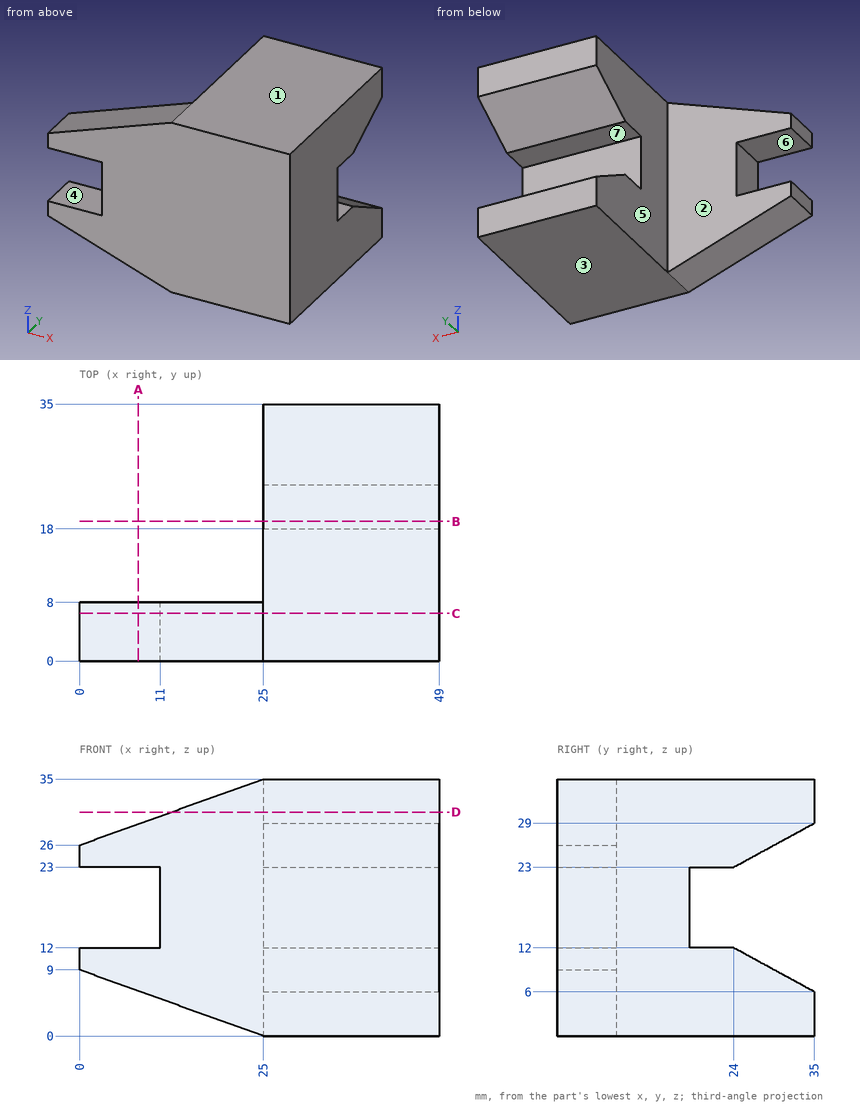
The drawing under review shows one solid part. Ordinate dimensions are in mm from its lowest x, y, z. A direction names the side the tool comes from. Coordinates: 2 decimals unless noted, no trailing zeros. Loops run counter-clockwise (first coordinate to the right, second up) from the corner with the lowest first, then second, coordinate; pieces in that order, holes last.
Item 1: Wall thickness on L1, parallel to Z at x = 30, y = 19; L2, parallel to Y at x = 9, z = 23.5; L3, parallel to X at y = 11.5, z = 2: over which ranges is each line inside the solid? List them lowest first.
Completed:
L1: z = 0 to 12, 23 to 35
L2: y = 0 to 8
L3: x = 25 to 49
Item 2: Add section C-C (y = 6.5). Write out the cut boundary in (x, z), and give its area (3 significant figures).
Completed:
outline: (0, 9) - (25, 0) - (49, 0) - (49, 35) - (25, 35) - (0, 26) - (0, 23) - (11, 23) - (11, 12) - (0, 12) - close
area: 1,370 mm2
Item 3: For the marked faces 5, 6 and 7, list the 3-axis set-ups (+Z, -Z, +X, -X, +Y, -Y) from which the entire face can be reached by the end or side of a thin tool; tool diameter is ignored.
Completed:
face 5: +Z, -Z, -X, +Y
face 6: -X, +Y, -Y
face 7: +X, -X, +Y
Item 4: Add section D-D (z = 30.5). Write out the cut boundary in (x, y).
Completed:
outline: (12.5, 0) - (49, 0) - (49, 35) - (25, 35) - (25, 8) - (12.5, 8) - close
Item 5: Clearance check with flat-ended pins moving along their axes: pin 1 (12 mm diameter, centred on y = 27.5, z = 20.5, fed in from -X); pin 2 (2 mm diameter, centred on x = 8.5, z = 23.5, fed in from +Y); pin 3 (12 mm diameter, centred on x = 40, z = 18.5, fed in from +Y). State where each tip first meets the part, or that it passes through.
Completed:
pin 1: stops at x = 25
pin 2: stops at y = 8
pin 3: stops at y = 26.75
Item 6: Add section A-A (x = 8). Write out the cut boundary in (y, z), and give its area (3 significant figures).
Completed:
outline: (0, 6.12) - (8, 6.12) - (8, 12) - (0, 12) - close; (0, 23) - (8, 23) - (8, 28.88) - (0, 28.88) - close
area: 94.1 mm2
Item 7: Add section B-B (y = 19). Write out the cut boundary in (x, z), and give its area (3 significant figures).
Completed:
outline: (25, 0) - (49, 0) - (49, 12) - (25, 12) - close; (25, 23) - (49, 23) - (49, 35) - (25, 35) - close
area: 576 mm2
Item 8: Draft analysis for pull direction Z (two halves, no side actions). For the marked faces 1, 2, 3 and 4, state which applies: pulls with the +Z half, pulls with the -Z half, needs draft (parallel to the pull), parting line crosses it, or undercut.
Completed:
face 1: pulls with the +Z half
face 2: needs draft
face 3: pulls with the -Z half
face 4: undercut
